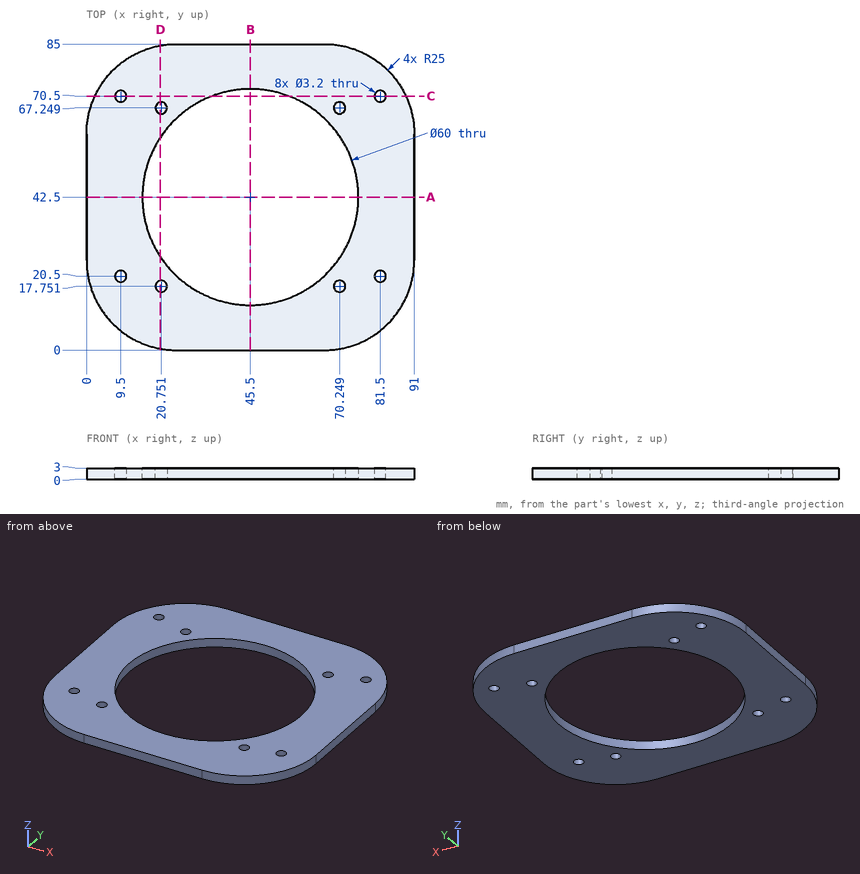
For this review, use the dimensioned drawing (mm, ordinates from the lowest corner) and the shaded views. Coordinates: 2 decimals unless noted, no trailing zeros. Write each loop counter-clockwise with the first axis right and the second up, starting at its lowest first coordinate (ties: lowest second). Pieces come first, ordered by that corner, then holes. Notation, with made-up numbers: (-22, -22.5) - (-6, -22.5) arc R15 ccw to (-6, 1.5) - close; hole circle Ø6 at (28, -35). An arc over 180 degrees is marked (long way). Answer as a JSON object with one key per item and string values. Group by question number.
1. Add section C-C (y = 70.5). Give the boundary of the cut face in (x, z), plus the area to 3 significant figures.
2. Add section A-A (y = 42.5). Give the boundary of the cut face in (x, z).
3. Add section B-B (x = 45.5). Give the boundary of the cut face in (y, z).
4. Clearance check with flat-ended pins moving along their axes: pin 1 Ø4 at (x, y) = (70.25, 17.75) entering from -Z; pin 2 Ø1 at (x, z) = (73, 1) entering from +Y. State where each tip first meets the part, or that it passes through.
5. To check wall thickness, follow probe 1 along Y at (x, z) = (22, 2.65); probe 2 along Y at (x, z) = (81.5, 1.1) (1 decimal); probe 3 along Y at (x, z) = (54, 1.1). State the ranges of each line that lie inside material, in increasing order.
6. Add section D-D (x = 20.5). Give the boundary of the cut face in (y, z), plus the area to 3 significant figures.
Findings:
{
 "1": {"outline": "(2.31, 0) - (7.9, 0) - (7.9, 3) - (2.31, 3) - close; (11.1, 0) - (34.73, 0) - (34.73, 3) - (11.1, 3) - close; (56.27, 0) - (79.9, 0) - (79.9, 3) - (56.27, 3) - close; (83.1, 0) - (88.69, 0) - (88.69, 3) - (83.1, 3) - close", "area": "175 mm²"},
 "2": {"outline": "(0, 0) - (15.5, 0) - (15.5, 3) - (0, 3) - close; (75.5, 0) - (91, 0) - (91, 3) - (75.5, 3) - close"},
 "3": {"outline": "(0, 0) - (12.5, 0) - (12.5, 3) - (0, 3) - close; (72.5, 0) - (85, 0) - (85, 3) - (72.5, 3) - close"},
 "4": {"pin 1": "z = 0", "pin 2": "y = 84.14"},
 "5": {"probe 1": "0.18 to 16.75, 18.75 to 23.85, 61.15 to 66.25, 68.25 to 84.82", "probe 2": "5.4 to 18.9, 22.1 to 68.9, 72.1 to 79.6", "probe 3": "0 to 13.73, 71.27 to 85"},
 "6": {"outline": "(0.41, 0) - (16.17, 0) - (16.17, 3) - (0.41, 3) - close; (19.33, 0) - (25.92, 0) - (25.92, 3) - (19.33, 3) - close; (59.08, 0) - (65.67, 0) - (65.67, 3) - (59.08, 3) - close; (68.83, 0) - (84.59, 0) - (84.59, 3) - (68.83, 3) - close", "area": "134 mm²"}
}
